Input: part model. Units: mm. Frame: model coordinates. Face numbers are marked on the shaded views. A direction names the side the tool comes from. Coordinates: 2 decimals unless noted, no trailing zeros. Order: outer loops, then holes, each group sorted by start corner. A loop starts at its lowest first (then second) coordinate and runs counter-clockwise, first axis right, second up. Notation, with made-up numbers: (2.5, 10) -> (22.5, 10) arc R22 cw to (22.5, 18) -> close; hole circle Ø5 at (80, 46.25). An arc over 180 degrees is marked (long way). Write each question's results on one line, items separated by ' | '.
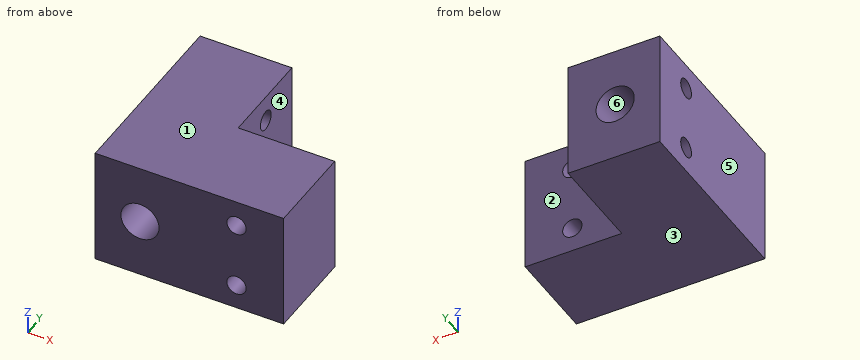
```python
from build123d import *

# Parameters (mm, degrees)
F1_DEPTH = 25
F2_R     = 2.05
F2_R_2   = 4.05
F3_DEPTH = 45
F4_R     = 2.05
F5_DEPTH = 25


with BuildPart() as f1:
    # F0 (on Top) → F1 (new body)
    with BuildSketch(Plane.XY):
        Polygon((0, 20.5), (-19.5, 20.5), (-19.5, -19.5), (20.5, -19.5), (20.5, 0), (0, 0), align=None)
    extrude(amount=F1_DEPTH)

    # F2 (on face) → F3 (cut)
    with BuildSketch(Plane.XZ.offset(19.5)):
        with Locations((10.5, 19.445103)):
            Circle(F2_R)
        with Locations((10.5, 5.321864)):
            Circle(F2_R)
        with Locations((-10, 12.5)):
            Circle(F2_R_2)
    extrude(amount=-F3_DEPTH, mode=Mode.SUBTRACT)

    # F4 (on face) → F5 (cut)
    with BuildSketch(Plane(origin=(-19.5, 0, 0), x_dir=(0, -1, 0), z_dir=(-1, 0, 0))):
        with Locations((-10.5, 19.5)):
            Circle(F4_R)
        with Locations((-10.5, 5.5)):
            Circle(F4_R)
    extrude(amount=-F5_DEPTH, mode=Mode.SUBTRACT)


solid = f1.part
```
(1) Cut plane B-B, the plane y = 10.5. Return loops of the section in (x, z), plus the area to 3 significant figures.
Return value:
outline: (-19.5, 0) -> (0, 0) -> (0, 3.45) -> (-19.5, 3.45) -> close; (-19.5, 7.55) -> (0, 7.55) -> (0, 17.45) -> (-19.5, 17.45) -> close; (-19.5, 21.55) -> (0, 21.55) -> (0, 25) -> (-19.5, 25) -> close; hole circle Ø8.1 at (-10, 12.5) | area: 276 mm2
(2) Pin query (flat end, axial travel): P1, Ø3.5, axis at x = 10.5, z = 5.32, coming from the -Y side; P2, Ø6, axis at x = 10.5, z = 6.5, coming from the +Y side. Return the tip coordinate at first contact, or that it passes through.
Return value:
P1: through | P2: y = 0
(3) Cut plane A-A, the plane x = -10. Return loops of the section in (y, z).
Return value:
outline: (-19.5, 0) -> (20.5, 0) -> (20.5, 8.45) -> (-19.5, 8.45) -> close; (-19.5, 16.55) -> (20.5, 16.55) -> (20.5, 25) -> (-19.5, 25) -> close; hole circle Ø4.1 at (10.5, 5.5); hole circle Ø4.1 at (10.5, 19.5)
(4) Reachability of the marked faces 1 and 2 from +Z, -Z, +X, -X, +Y, -Y: full face, straight path, thin tool, end or side. Return the list, or none.
Return value:
face 1: +Z, +X, -X, +Y, -Y | face 2: +Z, -Z, +X, +Y
(5) Mould query, pull axis X, two halves, no side actions, for the marked faces 3, 4, 5 and 6. Classes: +X half, -X half, draft (parallel to the pull), parting line (faces both ways), or undercut.
Return value:
face 3: draft | face 4: +X half | face 5: -X half | face 6: undercut
(6) Cut plane C-C, the plane z = 15.25. Return loops of the section in (x, y), plus the area to 3 significant figures.
Return value:
outline: (-19.5, -19.5) -> (-12.97, -19.5) -> (-12.97, 20.5) -> (-19.5, 20.5) -> close; (-7.03, -19.5) -> (20.5, -19.5) -> (20.5, 0) -> (0, 0) -> (0, 20.5) -> (-7.03, 20.5) -> close | area: 942 mm2
(7) Line query: line 1 along Z through (x, y) = (10.5, -10); line 2 along Z through (x, y) = (-10, 12); line 3 along Z through (x, y) = (10, -14). Output: solid intervals per line, ascending. Write a range as from..to.
Return value:
line 1: 0..3.27, 7.37..17.4, 21.5..25 | line 2: 0..4.1, 6.9..8.45, 16.55..18.1, 20.9..25 | line 3: 0..3.33, 7.31..17.46, 21.43..25
(8) Cut plane D-D, the plane x = -0.5. Return loops of the section in (y, z).
Return value:
outline: (-19.5, 0) -> (20.5, 0) -> (20.5, 25) -> (-19.5, 25) -> close; hole circle Ø4.1 at (10.5, 5.5); hole circle Ø4.1 at (10.5, 19.5)
